```python
from build123d import *

# Parameters (mm, degrees)
SKETCH1_R               = 11.5
BOSS_EXTRUDE1_DEPTH     = 130
CHAMFER1_SIZE           = 5
CUT_EXTRUDE1_DEPTH      = 132.013358098
CUT_EXTRUDE1_DEPTH_BACK = 132.013358098
SKETCH2_R               = 5


with BuildPart() as part:
    # Sketch1 → Boss-Extrude1 (new body)
    with BuildSketch(Plane.XY):
        Circle(SKETCH1_R)
    extrude(amount=BOSS_EXTRUDE1_DEPTH)

    # Chamfer1
    chamfer1_edges = [part.edges().sort_by_distance(p)[0] for p in [
        (-11.5, 0, 130),
    ]]
    chamfer(chamfer1_edges, length=CHAMFER1_SIZE)

    # Sketch2 → Cut-Extrude1 (cut, two sides: drawn at the far end of the back side and taken through both)
    with BuildSketch(Plane(origin=(0, 0, 0), x_dir=(1, 0, 0), z_dir=(0, 1, 0)).offset(-CUT_EXTRUDE1_DEPTH_BACK)):
        with Locations(Location((0, -15, 0), (0, 0, 270))):
            Circle(SKETCH2_R)
    extrude(amount=CUT_EXTRUDE1_DEPTH + CUT_EXTRUDE1_DEPTH_BACK, mode=Mode.SUBTRACT)


solid = part.part
```
Build history of the part. All positions in model axes, mm. Coordinates: 2 decimals unless noted, no trailing zeros. Write each loop counter-clockwise with the first axis right and the second up, starting at its lowest first coordinate (ties: lowest second). Pieces come first, ordered by that corner, then holes.
1. Drill centre lines: probe 1 along Z at (x, y) = (0, -5.5); probe 2 along X at (y, z) = (2.5, 15); probe 3 along X at (y, z) = (6.25, 15). Where is each one in solid material? Low to high.
Answer block:
probe 1: z = 0 to 10, 20 to 130
probe 2: x = -11.22 to -5, 5 to 11.22
probe 3: x = -9.65 to -5, 5 to 9.65
2. Band-saw the part on B-B, the plane x = 0. Give the cut face in (y, z).
Answer block:
outline: (-11.5, 0) - (11.5, 0) - (11.5, 10) - (-11.5, 10) - close; (-11.5, 20) - (11.5, 20) - (11.5, 125) - (6.5, 130) - (-6.5, 130) - (-11.5, 125) - close
3. Band-saw the part on D-D, the plane z = 15. Give the cut face in (x, y).
Answer block:
outline: (-5, -10.36) - (-5, 10.36) arc R11.5 ccw to start; (5, -10.36) arc R11.5 ccw to (5, 10.36) - close
4. Band-saw the part on C-C, the plane z = 35. Give the cut face in (x, y), and give its area (3 significant figures).
Answer block:
outline: circle Ø23 at (0, 0)
area: 415 mm2
5. Pull direction X, two halves, no side cores. Call faces 1 (the cylindrical face through (-4.436, -0.161, 17.307)), 2 (the conical face through (-5.35, -4.1, 129.76)), 3 (the flat face through (0, 0, 130)): released by +X, released by -X, zero draft, split by the parting line, or undercut.
Answer block:
face 1: undercut
face 2: split by the parting line
face 3: zero draft
6. Drop flat-ended pins along their axis: pin 1 (2 mm diameter, centred on x = 7.5, z = 56.5, fed in from +Y); pin 2 (1 mm diameter, centred on y = 5.5, z = 59, fed in from -X); pin 3 (10 mm diameter, centred on y = -9, z = 69.5, fed in from -X). Give the stop position or say it passes through.
Answer block:
pin 1: stops at y = 9.49
pin 2: stops at x = -10.36
pin 3: stops at x = -10.78
7. Band-saw the part on A-A, the plane y = 0. Give the cut face in (x, z).
Answer block:
outline: (-11.5, 0) - (11.5, 0) - (11.5, 125) - (6.5, 130) - (-6.5, 130) - (-11.5, 125) - close; hole circle Ø10 at (0, 15)
